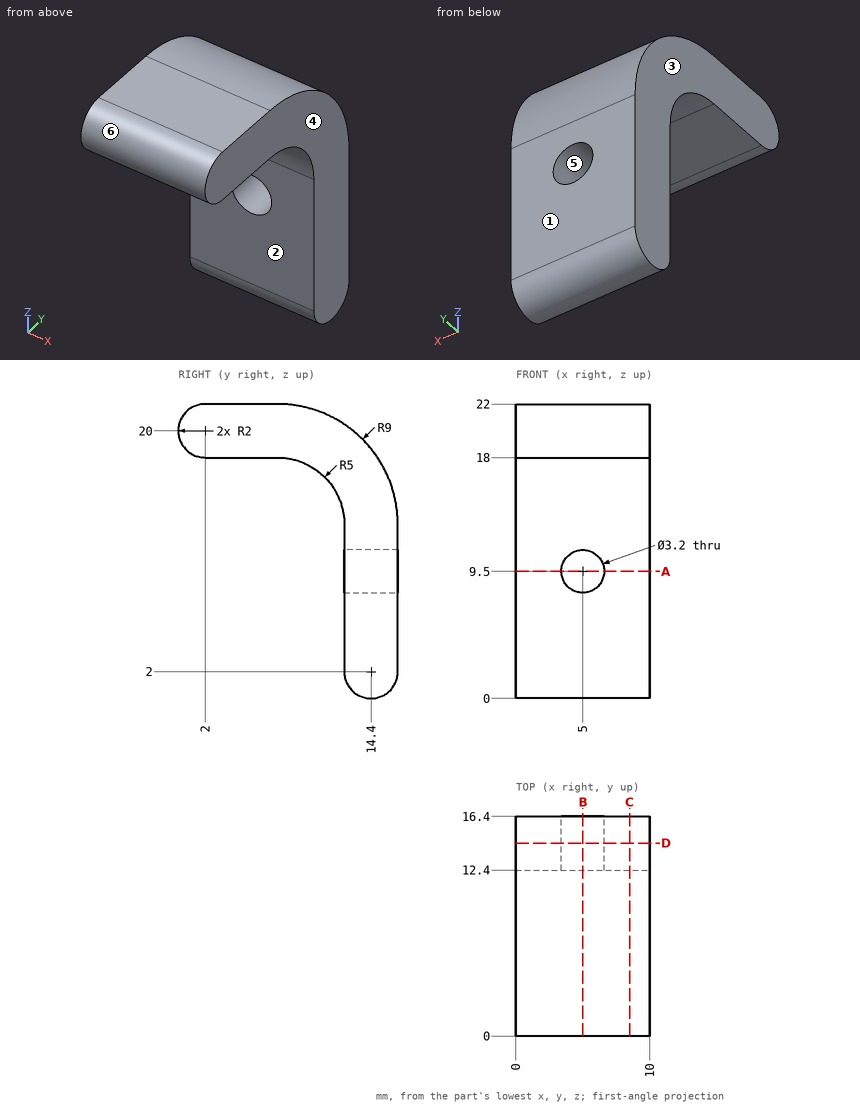
Can you work these out from the drawing? Everything is in mm from the part's minimum corner. A direction names the side the tool comes from. Round coordinates to 2 decimals unless told otherwise and drop trailing zeros. Loops run counter-clockwise (first coordinate to the right, second up) from the corner with the lowest first, then second, coordinate; pieces in that order, holes last. Notation, with made-up numbers: (-36, 19) - (-3, 19) arc R31 cw to (-3, 49) - close; hole circle Ø11 at (32, -6.75). An arc over 180 degrees is marked (long way). Answer in a Markdown table with one row per item. Add a question column.
(1) If we section it at B-B (x = 5): Please give me the cut outline in (y, z), plus the area to 3 significant figures.
(2) I'm going to push flat-ended pins straight in: pin 1 (4.5 mm diameter, centred on x = 5, y = 6, fed in from -Z); pin 2 (4 mm diameter, centred on x = 5, z = 15.5, fed in from -Y); pin 3 (3 mm diameter, centred on x = 2, y = 4.5, fed in from -Z). Where does each tip first touch, or does it pass through?
(3) If we section it at A-A (z = 9.5): Please give me the cut outline in (x, y).
(4) I need wall thicknesses on line 1 along X through (y, z) = (14, 9.5); line 2 along Z through (x, y) = (2.5, 6); line 3 along Y through (x, z) = (7.5, 8.5). Which ranges of each line are inside material? Lowest first, please.
(5) For the marked faces 1 and 2, which set-ups out of +Z, -Z, +X, -X, +Y, -Y let a thin tool reach every point of the face, with its end or its side?
(6) If we mould it in two halves opening along X, with no side actions, what happens to the marked faces 3, 4, 5 and 6? For each: pulls with the +X half, pulls with the -X half, needs draft (parallel to the pull), parting line crosses it, or undercut.
(7) If we section it at D-D (y = 14.4): Please give me the cut outline in (x, z), plus the area to 3 significant figures.
(8) If we section it at C-C (x = 8.5): Please give me the cut outline in (y, z).
Model answer:
| question | item | result |
|---|---|---|
| 1 | outline | (2, 18) - (7.4, 18) arc R5 cw to (12.4, 13) - (12.4, 11.1) - (16.4, 11.1) - (16.4, 13) arc R9 ccw to (7.4, 22) - (2, 22) arc R2 ccw to start; (12.4, 2) arc R2 ccw to (16.4, 2) - (16.4, 7.9) - (12.4, 7.9) - close |
| 1 | area | 109 mm² |
| 2 | pin 1 | stops at z = 17.93 |
| 2 | pin 2 | stops at y = 9.58 |
| 2 | pin 3 | stops at z = 18 |
| 3 | outline | (0, 12.4) - (3.4, 12.4) - (3.4, 16.4) - (0, 16.4) - close; (6.6, 12.4) - (10, 12.4) - (10, 16.4) - (6.6, 16.4) - close |
| 4 | line 1 | x = 0 to 3.4, 6.6 to 10 |
| 4 | line 2 | z = 18 to 22 |
| 4 | line 3 | y = 12.4 to 16.4 |
| 5 | face 1 | +Z, -Z, +X, -X, +Y |
| 5 | face 2 | -Z, +X, -X, -Y |
| 6 | face 3 | pulls with the -X half |
| 6 | face 4 | pulls with the +X half |
| 6 | face 5 | undercut |
| 6 | face 6 | needs draft |
| 7 | outline | (0, 0) - (10, 0) - (10, 18.66) - (0, 18.66) - close; hole circle Ø3.2 at (5, 9.5) |
| 7 | area | 179 mm² |
| 8 | outline | (2, 18) - (7.4, 18) arc R5 cw to (12.4, 13) - (12.4, 2) arc R2 ccw to (16.4, 2) - (16.4, 13) arc R9 ccw to (7.4, 22) - (2, 22) arc R2 ccw to start |
